Part model, mm, in its own coordinate system. A direction names the side the tool comes from. Give positions to 0.01 mm unless a question says otherwise; leave off trailing zeros. Order: outer loops, then holes, each group sorted by start corner. A loop starts at its lowest first (then second) coordinate and runs counter-clockwise, first axis right, second up. Notation, with made-up numbers: M -32,-39.75 L 15,-39.75 A26 cw 15,-17.75 Z; hole C 71.5,12.25 d11. An arc over 180 degrees is marked long. Return JSON: item names as keys, results as strings.
from build123d import *

# Parameters (mm, degrees)
F0_W     = 180
F0_H     = 180
F0_W_2   = 130
F0_H_2   = 130
F1_DEPTH = 4
F2_W     = 180
F2_H     = 180
F2_W_2   = 160.5
F2_H_2   = 160.5
F3_DEPTH = 1


with BuildPart() as f1:
    # F0 (on Top) → F1 (new body)
    with BuildSketch(Plane.XY):
        with Locations((-3.792722, 36.59609)):
            Rectangle(F0_W, F0_H)
        with Locations((-3.792722, 36.59609)):
            Rectangle(F0_W_2, F0_H_2, mode=Mode.SUBTRACT)
    extrude(amount=F1_DEPTH)

    # F2 (on face) → F3 (join)
    with BuildSketch(Plane.XY.offset(4)):
        with Locations((-3.792722, 36.59609)):
            Rectangle(F2_W, F2_H)
        with Locations((-4.292722, 37.09609)):
            Rectangle(F2_W_2, F2_H_2, mode=Mode.SUBTRACT)
    extrude(amount=F3_DEPTH)


solid = f1.part
Q1. Band-saw the part on B-B (z = 1.8). Give the cut face in (x, y), then the cut area to 3 significant figures.
Established:
{"outline": "M -93.79,-53.4 L 86.21,-53.4 L 86.21,126.6 L -93.79,126.6 Z; hole M -68.79,-28.4 L 61.21,-28.4 L 61.21,101.6 L -68.79,101.6 Z", "area": "15,500 mm²"}
Q2. Two-plate mould, pull along Y, no slides. Class faces 1 (the flat face through (-5, 101.596, 2)), 2 (the flat face through (-5, -53.404, 2)), 3 (the flat face through (86.207, 35, 2)): +Y half, -Y half, draft (parallel to the pull), parting line (faces both ways), or undercut.
Established:
{"face 1": "undercut", "face 2": "-Y half", "face 3": "draft"}
Q3. 3-axis set-ups, long thin cutter, end or side, ignore diameter. For faces 4 (the flat face through (-77, 38, 4)), 5 (the flat face through (75, 38, 0)), 6 (the flat face through (-5, -28.404, 2)): which of +Z, -Z, +X, -X, +Y, -Y reach the whole face in a straight line?
Established:
{"face 4": "+Z", "face 5": "-Z, +X, -X, +Y, -Y", "face 6": "+Z, -Z"}
Q4. Pin check, flat tip, straight feed: pin 1 (6 mm diameter, centred on x = 13, y = 106.5, fed in from -Z). Stop position of the tip, or through.
Established:
{"pin 1": "stops at z = 0"}
Q5. Band-saw the part on D-D (x = -76.5). Give the cut face in (y, z).
Established:
{"outline": "M -53.4,0 L 126.6,0 L 126.6,5 L 117.35,5 L 117.35,4 L -43.15,4 L -43.15,5 L -53.4,5 Z"}
Q6. Band-saw the part on C-C (y = 12.5). Give the cut face in (x, z), then the cut area to 4 significant figures.
Established:
{"outline": "M -93.79,0 L -68.79,0 L -68.79,4 L -84.54,4 L -84.54,5 L -93.79,5 Z; M 61.21,0 L 86.21,0 L 86.21,5 L 75.96,5 L 75.96,4 L 61.21,4 Z", "area": "219.5 mm²"}
Q7. Band-saw the part on A-A (x = -9.5). Give the cut face in (y, z).
Established:
{"outline": "M -53.4,0 L -28.4,0 L -28.4,4 L -43.15,4 L -43.15,5 L -53.4,5 Z; M 101.6,0 L 126.6,0 L 126.6,5 L 117.35,5 L 117.35,4 L 101.6,4 Z"}
Q8. Probe line 1 along X through (y, z) = (91, 4.5); line 2 along Y through (x, z) = (-41.5, 0.5); line 3 along Y through (x, z) = (30, 4.55). List the from-to ranges inside material, lowest first.
Established:
{"line 1": "x = -93.79 to -84.54, 75.96 to 86.21", "line 2": "y = -53.4 to -28.4, 101.6 to 126.6", "line 3": "y = -53.4 to -43.15, 117.35 to 126.6"}
